Could you check a few things on this drawing? It's one solid part, dimensions in mm from its lowest x, y, z. A direction names the side the tool comes from. Give positions to 0.01 mm unless a question says otherwise; leave off trailing zeros. Loops run counter-clockwise (first coordinate to the right, second up) from the corner with the lowest first, then second, coordinate; pieces in that order, holes last. Notation, with made-up numbers: (50, 2) -> (90, 2) arc R19 cw to (90, 20) -> close; hole circle Ø10 at (61, 11). An arc over 180 degrees is marked (long way). One line per question, with ' | ' between items.
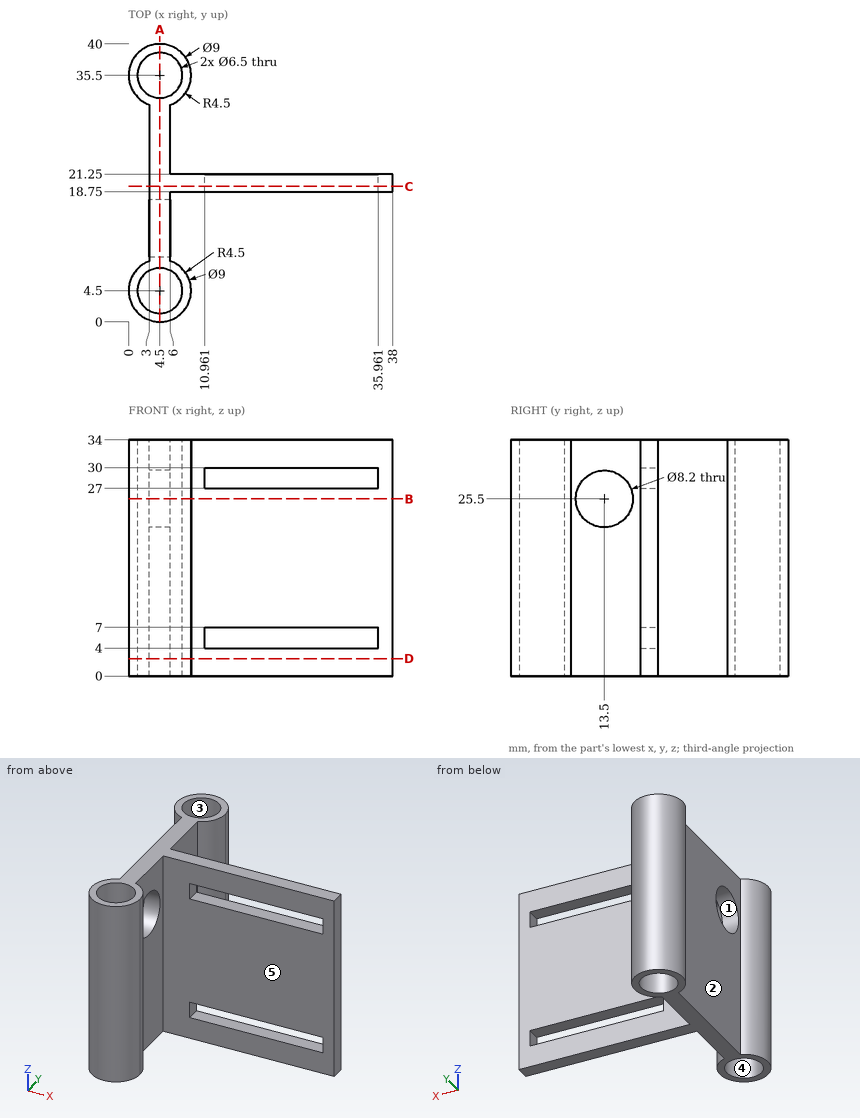
Q1. If we section it at A-A (x = 4.5): Write out the boundary of the cut face in (y, z).
Entries:
outline: (0, 0) -> (1.25, 0) -> (1.25, 34) -> (0, 34) -> close; (7.75, 0) -> (32.25, 0) -> (32.25, 34) -> (7.75, 34) -> close; (38.75, 0) -> (40, 0) -> (40, 34) -> (38.75, 34) -> close; hole circle Ø8.2 at (13.5, 25.5)
Q2. On a 3-axis mill with a long thin cutter (end or side, diameter ignored), from which of +Z, -Z, +X, -X, +Y, -Y can I reach the whole of each face in a straight line? I mean the marked faces 4 and 5. Say none if no direction works.
Entries:
face 4: +Z, -Z | face 5: +Z, -Z, +X
Q3. If I drill on probe 1 along Y at (x, z) = (4, 25); probe 2 along Y at (x, z) = (9.5, 28.5); probe 3 along X at (y, z) = (29.5, 17.5), over which ranges is the centre line in solid material (lowest first)? Write a range as from..to.
Entries:
probe 1: 0.03..1.29, 7.71..9.43, 17.57..32.29, 38.71..39.97 | probe 2: 18.75..21.25 | probe 3: 3..6
Q4. For pin 1 Ø6 at (x, z) = (23.5, 8.5) entering from +Y; pin 2 Ø2 at (y, z) = (19.5, 28.5) entering from -X; pin 3 Ø1 at (x, z) = (12.5, 26.5) entering from -Y; pin 4 Ø5 at (x, y) = (4.5, 4.5) entering from -Z, each with a flat end and sliding along its axis, tell me the tip position at first contact or that it passes through.
Entries:
pin 1: y = 21.25 | pin 2: x = 3 | pin 3: y = 18.75 | pin 4: through
Q5. If we section it at C-C (y = 19.5): Write out the boundary of the cut face in (x, z), plus the area to 3 significant figures.
Entries:
outline: (3, 0) -> (38, 0) -> (38, 34) -> (3, 34) -> close; hole (10.96, 4) -> (35.96, 4) -> (35.96, 7) -> (10.96, 7) -> close; hole (10.96, 27) -> (35.96, 27) -> (35.96, 30) -> (10.96, 30) -> close | area: 1,040 mm²
Q6. If we section it at B-B (z = 25.5): Write out the boundary of the cut face in (x, y).
Entries:
outline: (3, 8.74) arc R4.5 ccw (long way) to (9, 4.5) arc R4.5 ccw to (6, 8.74) -> (6, 9.4) -> (3, 9.4) -> close; (3, 17.6) -> (6, 17.6) -> (6, 18.75) -> (38, 18.75) -> (38, 21.25) -> (6, 21.25) -> (6, 31.26) arc R4.5 ccw to (9, 35.5) arc R4.5 ccw (long way) to (3, 31.26) -> close; hole circle Ø6.5 at (4.5, 4.5); hole circle Ø6.5 at (4.5, 35.5)
Q7. If we section it at D-D (z = 2.5): Write out the boundary of the cut face in (x, y).
Entries:
outline: (3, 8.74) arc R4.5 ccw (long way) to (9, 4.5) arc R4.5 ccw to (6, 8.74) -> (6, 18.75) -> (38, 18.75) -> (38, 21.25) -> (6, 21.25) -> (6, 31.26) arc R4.5 ccw to (9, 35.5) arc R4.5 ccw (long way) to (3, 31.26) -> close; hole circle Ø6.5 at (4.5, 4.5); hole circle Ø6.5 at (4.5, 35.5)
Q8. If we mould it in two halves opening along X, with no side actions, what happens to the marked faces 1, 2 and 3? For each: pulls with the +X half, pulls with the -X half, needs draft (parallel to the pull), parting line crosses it, or undercut.
Entries:
face 1: needs draft | face 2: pulls with the -X half | face 3: undercut
